Design review of the part shown in the three views and the two pictorial views. Dimensions are in mm from the part's minimum x, y and z. Give positions to 0.01 mm unless a question says otherwise; leave off trailing zeros. Write each loop counter-clockwise with the first axis right and the second up, starting at its lowest first coordinate (ties: lowest second). Pieces come first, ordered by that corner, then holes.
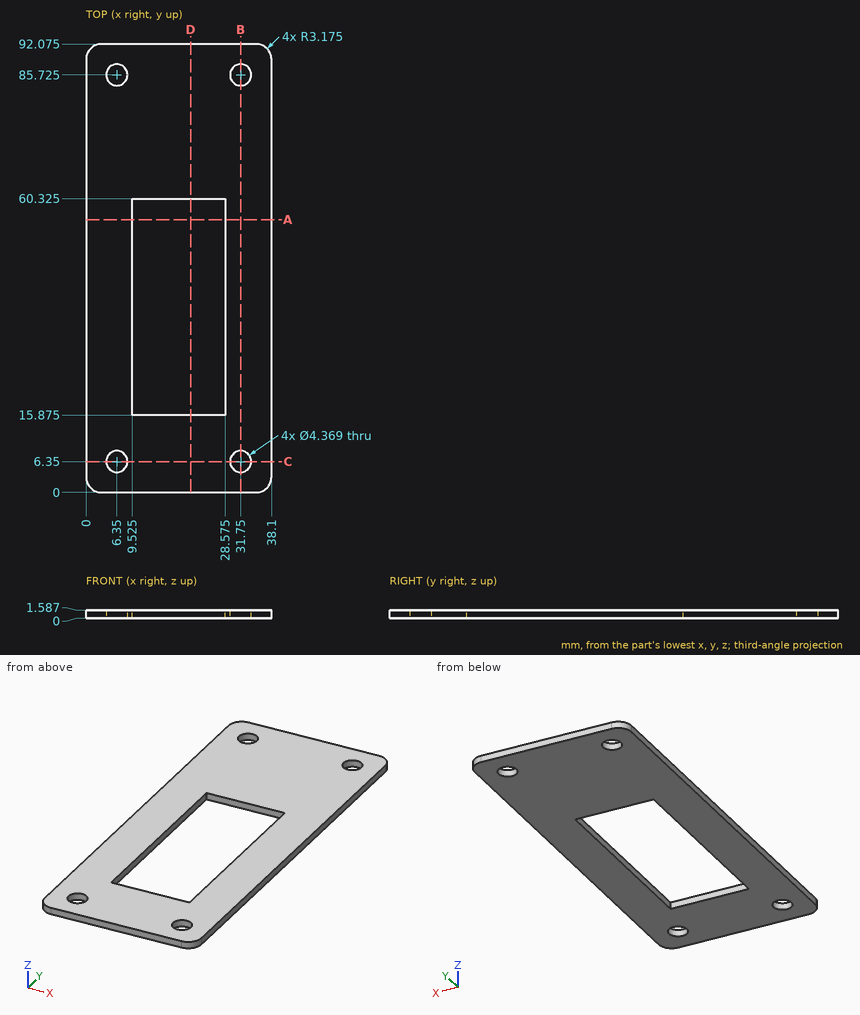
(1) Consider section C-C, the plane y = 6.35. Give the boundary of the cut face in (x, z) (1 decimal).
Resolved:
outline: (0, 0) - (4.2, 0) - (4.2, 1.6) - (0, 1.6) - close; (8.5, 0) - (29.6, 0) - (29.6, 1.6) - (8.5, 1.6) - close; (33.9, 0) - (38.1, 0) - (38.1, 1.6) - (33.9, 1.6) - close
(2) Consider section A-A, the plane y = 56. Give the boundary of the cut face in (x, z) (1 decimal).
Resolved:
outline: (0, 0) - (9.5, 0) - (9.5, 1.6) - (0, 1.6) - close; (28.6, 0) - (38.1, 0) - (38.1, 1.6) - (28.6, 1.6) - close
(3) Clearance check with a flat-ended pin moving along its axis: P1, Ø4, axis at x = 31.75, y = 85.725, coming from the -Z side. State where the tip first meets the part, or that it passes through.
Resolved:
P1: passes through
(4) To check wall thickness, follow L1, parallel to Y at x = 6.35, z = 1.1 (1 decimal); L2, parallel to X at y = 86, z = 0.55; L3, parallel to Y at x = 8, z = 0.35 (1 decimal). State the ranges of each line that lie inside material, in increasing order.
Resolved:
L1: y = 0 to 4.2, 8.5 to 83.5, 87.9 to 92.1
L2: x = 0 to 4.18, 8.52 to 29.58, 33.92 to 38.1
L3: y = 0 to 4.9, 7.8 to 84.3, 87.2 to 92.1
(5) Consider section B-B, the plane x = 31.75. Give the boundary of the cut face in (y, z) (1 decimal), then the cut area to 3 significant figures.
Resolved:
outline: (0, 0) - (4.2, 0) - (4.2, 1.6) - (0, 1.6) - close; (8.5, 0) - (83.5, 0) - (83.5, 1.6) - (8.5, 1.6) - close; (87.9, 0) - (92.1, 0) - (92.1, 1.6) - (87.9, 1.6) - close
area: 132 mm2
(6) Consider section D-D, the plane x = 21.5. Give the boundary of the cut face in (y, z) (1 decimal).
Resolved:
outline: (0, 0) - (15.9, 0) - (15.9, 1.6) - (0, 1.6) - close; (60.3, 0) - (92.1, 0) - (92.1, 1.6) - (60.3, 1.6) - close
